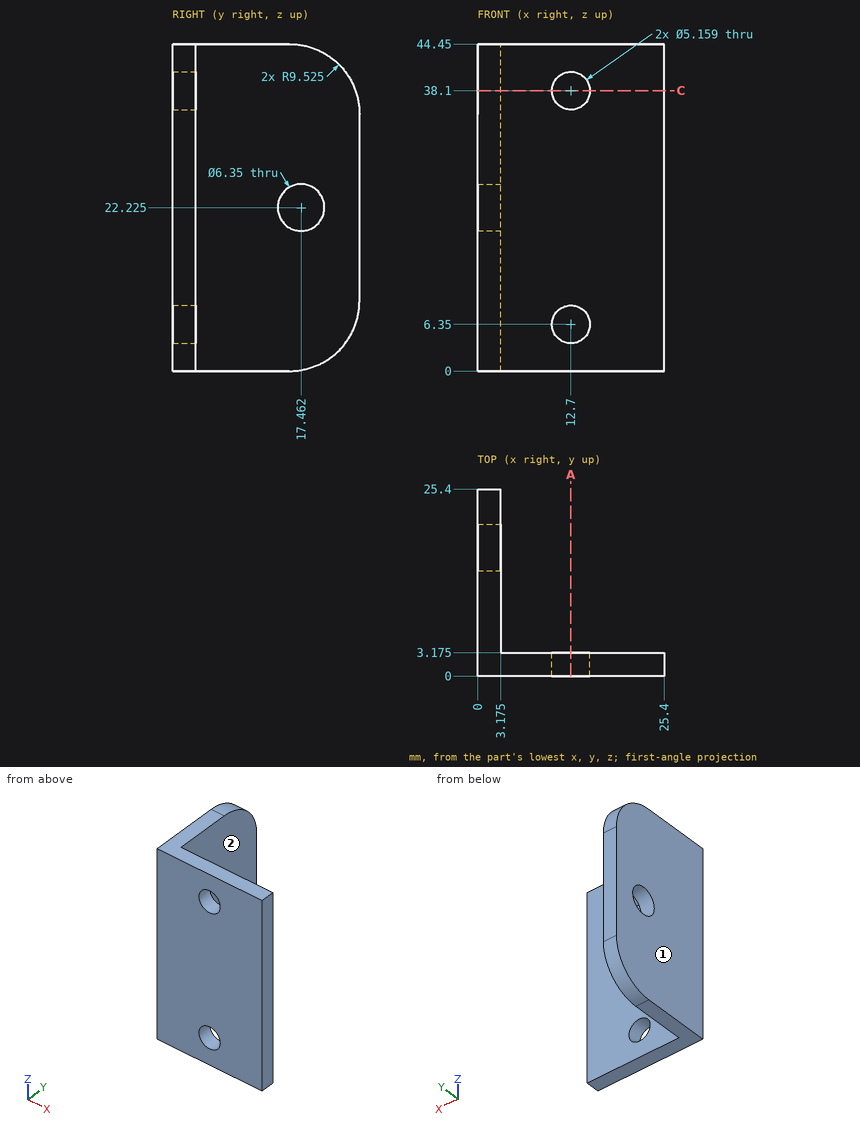
Print and shaded views of the part. All mm, measured from the part's lowest x, y and z. A direction names the side the tool comes from. Round coordinates to 2 decimals unless told otherwise and drop trailing zeros. Write each loop counter-clockwise with the first axis right and the second up, starting at its lowest first coordinate (ties: lowest second). Pieces come first, ordered by that corner, then holes. Notation, with made-up numbers: M -18,-32.75 L 28,-32.75 A12 ccw 28,-25.75 Z; hole C -35,15.25 d4. An arc over 180 degrees is marked long. One line per question, with ' | ' between items.
(1) Probe line 1 along Z through (x, y) = (12.7, 0.75); line 2 along X through (y, z) = (1.6, 38.1); line 3 along X through (y, z) = (4.25, 4) (1 decimal). List the from-to ranges inside material, lowest first.
Answer key:
line 1: z = 0 to 3.77, 8.93 to 35.52, 40.68 to 44.45 | line 2: x = 0 to 10.12, 15.28 to 25.4 | line 3: x = 0 to 3.2
(2) Pin check, flat tips, straight feed: pin 1 (11 mm diameter, centred on y = 11.5, z = 14.5, fed in from +X) (1 decimal); pin 2 (10 mm diameter, centred on x = 16, z = 9.5, fed in from +Y) (1 decimal); pin 3 (2 mm diameter, centred on x = 4, z = 5.5, fed in from +Y); pin 4 (4 mm diameter, centred on y = 17.46, z = 22.22, fed in from -X). Stop position of each tip, or through.
Answer key:
pin 1: stops at x = 3.2 | pin 2: stops at y = 3.2 | pin 3: stops at y = 24.75 | pin 4: passes through
(3) Saw through at A-A on x = 12.7. Count the separate pieces of the cut face and the enclosed holes in it, then the cut area to 3 significant figures.
Answer key:
separate pieces: 3 | enclosed holes: 0 | area: 108 mm^2
(4) 3-axis set-ups, long thin cutter, end or side, ignore diameter. For the marked faces 1 and 2: which of +Z, -Z, +X, -X, +Y, -Y reach the whole face in a straight line?
Answer key:
face 1: +Z, -Z, -X, +Y, -Y | face 2: +Z, -Z, +X, +Y
(5) Saw through at C-C on z = 38.1. Write the cut outline in (x, y) (1 decimal).
Answer key:
outline: M 0,0 L 10.1,0 L 10.1,3.2 L 3.2,3.2 L 3.2,24.9 L 0,24.9 Z; M 15.3,0 L 25.4,0 L 25.4,3.2 L 15.3,3.2 Z
